Autodesk Inventor part; units mm, degrees
ref_plane "Work Plane1" through (0, 0, -28) normal (0, 0, -1) x (-1, 0, 0)
ref_plane "YZ Plane" through (0, 0, 0) normal (1, 0, 0) x (0, 1, 0)
ref_plane "XZ Plane" through (0, 0, 0) normal (0, 1, 0) x (-1, 0, 0)
sketch "Sketch2" plane through (0, 0, 0) normal (0, 0, 1) x (1, 0, 0)
  circle A0 centre (0, 0) radius 45
  dimension "d11" = 90
extrude "Extrusion2" add sketch "Sketch2" along normal blind 118
sketch "Sketch3" plane through (0, 0, 0) normal (0, 0, -1) x (-1, 0, 0)
  circle A0 centre (0, 0) radius 4
  dimension "d14" = 8
extrude "Extrusion3" add sketch "Sketch3" along normal blind 70
thread "Thread1"
sketch "Sketch4" plane through (0, 0, -70) normal (0, 0, -1) x (-1, 0, 0)
  line L0 (3.4641, 2) -> (-3.4641, 2)
  arc A0 (3.4641, 2) -> (-3.4641, 2) centre (0, 0) ccw
  circle A1 centre (0, 0) radius 4
  dimension "d19" = 2
extrude "Extrusion4" cut sketch "Sketch4" against normal blind 17 contours L0 A0
ref_plane "Work Plane1" through (0, 0, -28) normal (0, 0, -1) x (-1, 0, 0)
sketch "Sketch5" plane through (0, 0, -28) normal (0, 0, -1) x (-1, 0, 0)
  circle A0 centre (0, 0) radius 4
  circle A1 centre (0, 0) radius 5.5
  dimension "d23" = 1.5
extrude "Extrusion5" add sketch "Sketch5" against normal blind 1
sketch "Sketch6" plane through (0, 0, 0) normal (0, 0, -1) x (-1, 0, 0)
  circle A0 centre (0, 0) radius 26 construction
  point P0 (0, -26)
  point P1 (-26, 0)
  point P2 (0, 26)
  point P3 (26, 0)
  dimension "d26" = 52
hole "Hole1" at (0, -26, 0) at (26, 0, 0) at (0, 26, 0) at (-26, 0, 0) direction (0, 0, 1) diameter 3.242 depth 15 tip angle 118
sketch "Sketch7" plane through (0, 0, 0) normal (0, 1, 0) x (-1, 0, 0)
  circle A0 centre (0, 14.6614) radius 5
  point P0 (0, 0)
  dimension "d34" = 10
extrude "Extrusion6" add sketch "Sketch7" along normal blind 85
properties part number "P01 - Fan Motor" material "SAE 1020"
Check sheet for the modelled part. Datum: model origin and axes. Units: mm. A direction names the side the tool comes from. Give positions to 0.01 mm unless a question says otherwise; leave off trailing zeros. Write each loop counter-clockwise with the first axis right and the second up, starting at its lowest first coordinate (ties: lowest second). Pieces come first, ordered by that corner, then holes.
Item 1: Cross-section at B-B (x = -36.5). Enter the section's corners in (y, z), and give its area (3 significant figures).
Item 2: Cross-section at C-C (y = 56). Enter the section's corners in (x, z).
Item 3: Gauge pin test, flat ends, axial feed: pin 1 (2.5 mm diameter, centred on x = 0, y = 26, fed in from -Z); pin 2 (10 mm diameter, centred on x = 26.5, y = 0, fed in from -Z); pin 3 (1 mm diameter, centred on x = -1.5, y = 3, fed in from -Z); pin 4 (4 mm diameter, centred on x = -7.5, y = 60, fed in from +Z). Record the tip position at first contact, or that the pin passes through.
Item 4: Access from +Z, -Z, +X, -X, +Y, -Y to the whole of each face (thin tool, end or side, straight path). Record for faces 1 (the face through (0, 2, -62)), 2 (the face through (1.19, -5.37, -27.51)), 3 (the face through (4, -2, -27)).
Item 5: Cross-section at A-A (z = -40). Enter the section's corners in (x, y), and give its area (3 significant figures).
Item 6: Draft check along Z on faces 4 (the face through (0.867, 3.905, -13.311)), 5 (the face through (-1, 1, 118)), 6 (the face through (0.651, 64.578, 9.704)), 7 (the face through (0, 0, -70)). Enter one of: released by +Z, released by -Z, zero draft, split by the parting line, or undercut.
Item 7: Cross-section at D-D (x = 35). Enter the section's corners in (y, z).
Item 8: Scan lines: L1, parallel to Y at x = 0, z = 5; L2, parallel to Z at x = -14, y = 41; L3, parallel to Y at x = 1.5, z = 67.5 (3 decimals). Record each from-to range of solid material in increasing order.
Report:
1. outline: (-26.32, 0) - (26.32, 0) - (26.32, 118) - (-26.32, 118) - close
1. area: 6,210 mm2
2. outline: circle Ø10 at (0, 14.66)
3. pin 1: stops at z = 9.66
3. pin 2: stops at z = 0
3. pin 3: stops at z = -53
3. pin 4: passes through
4. face 1: -Z, +X, -X, +Y
4. face 2: -Z
4. face 3: none
5. outline: circle Ø8 at (0, 0)
5. area: 50.3 mm2
6. face 4: undercut
6. face 5: released by +Z
6. face 6: split by the parting line
6. face 7: released by -Z
7. outline: (-28.28, 0) - (28.28, 0) - (28.28, 118) - (-28.28, 118) - close
8. L1: y = -45 to -27.62, -24.38 to 24.38, 27.62 to 45
8. L2: z = 0 to 118
8. L3: y = -44.975 to 44.975
